```python
from build123d import *

# Parameters (mm, degrees)
SKETCH1_R           = 52.5
BOSS_EXTRUDE2_DEPTH = 2
SKETCH4_R           = 3.175
CUT_EXTRUDE2_DEPTH  = 2
SKETCH5_R           = 7.5
CUT_EXTRUDE3_DEPTH  = 102
SKETCH6_R           = 7.5
CUT_EXTRUDE4_DEPTH  = 102
SKETCH7_R           = 7.5
CUT_EXTRUDE5_DEPTH  = 102
SKETCH8_R           = 17.5
CUT_EXTRUDE6_DEPTH  = 10


with BuildPart() as part:
    # Sketch1 → Boss-Extrude2 (new body)
    with BuildSketch(Plane.XY):
        Circle(SKETCH1_R)
    extrude(amount=BOSS_EXTRUDE2_DEPTH)

    # Sketch4 → Cut-Extrude2 (cut)
    with BuildSketch(Plane.XY):
        with Locations((0, 21.5)):
            Circle(SKETCH4_R)
        with Locations((8.744837826, 19.641227339)):
            Circle(SKETCH4_R)
        with Locations((15.977613748, 14.386308037)):
            Circle(SKETCH4_R)
        with Locations((20.4477151, 6.643865379)):
            Circle(SKETCH4_R)
        with Locations((21.38222075, -2.24736196)):
            Circle(SKETCH4_R)
        with Locations((18.619546181, -10.75)):
            Circle(SKETCH4_R)
        with Locations((12.637382924, -17.393865379)):
            Circle(SKETCH4_R)
        with Locations((4.470101353, -21.030173416)):
            Circle(SKETCH4_R)
        with Locations((-4.470101353, -21.030173416)):
            Circle(SKETCH4_R)
        with Locations((-12.637382924, -17.393865379)):
            Circle(SKETCH4_R)
        with Locations((-18.619546181, -10.75)):
            Circle(SKETCH4_R)
        with Locations((-21.38222075, -2.24736196)):
            Circle(SKETCH4_R)
        with Locations((-20.4477151, 6.643865379)):
            Circle(SKETCH4_R)
        with Locations((-15.977613748, 14.386308037)):
            Circle(SKETCH4_R)
        with Locations((-8.744837826, 19.641227339)):
            Circle(SKETCH4_R)
    extrude(amount=CUT_EXTRUDE2_DEPTH, mode=Mode.SUBTRACT)

    # Sketch5 → Cut-Extrude3 (cut)
    with BuildSketch(Plane(origin=(-10.124934849, 0, 21.712992854), x_dir=(0, -1, 0), z_dir=(-0.4226182617407003, 0, 0.9063077870366496))):
        with Locations(Location((0, 37.5, 0), (0, 0, 270))):
            Circle(SKETCH5_R)
    extrude(amount=-CUT_EXTRUDE3_DEPTH, mode=Mode.SUBTRACT)

    # Sketch6 → Cut-Extrude4 (cut)
    with BuildSketch(Plane(origin=(6.212874781, 10.761014782, 26.647105929), x_dir=(0.86602540378444, -0.4999999999999977, 0), z_dir=(-0.21130913087034603, -0.36599815077066267, -0.9063077870366526))):
        with Locations(Location((0, 37.5, 0), (0, 0, 270))):
            Circle(SKETCH6_R)
    extrude(amount=CUT_EXTRUDE4_DEPTH, mode=Mode.SUBTRACT)

    # Sketch7 → Cut-Extrude5 (cut)
    with BuildSketch(Plane(origin=(6.212874781, -10.761014782, 26.647105929), x_dir=(0.8660254037844399, 0.4999999999999978, 0), z_dir=(0.2113091308703492, -0.36599815077066805, 0.9063077870366496))):
        with Locations(Location((0, 37.5, 0), (0, 0, 270))):
            Circle(SKETCH7_R)
    extrude(amount=-CUT_EXTRUDE5_DEPTH, mode=Mode.SUBTRACT)

    # Sketch8 → Cut-Extrude6 (cut)
    with BuildSketch(Plane.XY):
        Circle(SKETCH8_R)
    extrude(amount=CUT_EXTRUDE6_DEPTH, mode=Mode.SUBTRACT)


solid = part.part
```
Build history of the part. All positions in model axes, mm. Give positions to 0.01 mm unless a question says otherwise; leave off trailing zeros. Loops run counter-clockwise (first coordinate to the right, second up) from the corner with the lowest first, then second, coordinate; pieces in that order, holes last. Notation, with made-up numbers: (24.5, -37) -> (82.5, -37) arc R23 cw to (82.5, -16) -> close; hole circle Ø8 at (46, 67.25). An arc over 180 degrees is marked (long way). One line per question, with ' | ' between items. Start each with the question number.
1) Two-plate mould, pull along X, no slides. Class faces 1 (the cylindrical face through (-17.515, 5.428, 0.986)), 2 (the cylindrical face through (50.076, 15.77, 0.986)), 3 (the flat face through (-1, -23, 0)): released by +X, released by -X, zero draft, split by the parting line, or undercut.
2) Cut at A-A (x = 0). Give the cut face in (y, z) (3 decimals), plus the area to 3 significant figures.
3) Probe L1, parallel to Y at x = 10, z = 1.6; L2, parallel to Y at x = -24, z = 1.4; L3, parallel to Y at x = 8, z = 0.7. List the from-to ranges inside material, lowest first.
4) Cut at B-B (y = 21.5). Give the cut face in (x, z) (3 decimals), plus the area to 3 significant figures.
5) Cut at C-C (z = 0.65). Count the separate pieces of the cut face and the enclosed holes in it, plus the area to 3 significant figures.
6) Cut at D-D (y = -10.75). Give the cut face in (x, z).
Return value:
1) face 1: undercut | face 2: split by the parting line | face 3: zero draft
2) outline: (-52.5, 0) -> (-17.5, 0) -> (-17.5, 2) -> (-52.5, 2) -> close; (17.5, 0) -> (18.325, 0) -> (18.325, 2) -> (17.5, 2) -> close; (24.675, 0) -> (52.5, 0) -> (52.5, 2) -> (24.675, 2) -> close | area: 127 mm^2
3) L1: -51.54 to -19.16, -15.63 to -14.36, 14.36 to 16.72, 22.56 to 51.54 | L2: -46.69 to -42.7, -28.49 to -4.04, -0.45 to 28.49, 42.7 to 46.69 | L3: -51.89 to -15.56, 15.56 to 16.55, 22.73 to 51.89
4) outline: (-47.896, 0) -> (-11.319, 0) -> (-11.319, 2) -> (-47.896, 2) -> close; (-6.171, 0) -> (-3.175, 0) -> (-3.175, 2) -> (-6.171, 2) -> close; (3.175, 0) -> (6.171, 0) -> (6.171, 2) -> (3.175, 2) -> close; (11.319, 0) -> (47.896, 0) -> (47.896, 2) -> (11.319, 2) -> close | area: 158 mm^2
5) separate pieces: 1 | enclosed holes: 19 | area: 6,640 mm^2
6) outline: (-51.39, 0) -> (-21.79, 0) -> (-21.79, 2) -> (-51.39, 2) -> close; (-15.44, 0) -> (-13.81, 0) -> (-13.81, 2) -> (-15.44, 2) -> close; (13.81, 0) -> (15.44, 0) -> (15.44, 2) -> (13.81, 2) -> close; (21.79, 0) -> (51.39, 0) -> (51.39, 2) -> (21.79, 2) -> close
